Input: part model. Units: mm. Frame: model coordinates. Coordinates: 2 decimals unless noted, no trailing zeros. Write each loop counter-clockwise with the first axis right and the second up, starting at its lowest first coordinate (ties: lowest second). Pieces come first, ordered by that corner, then holes. Notation, with made-up numbers: M 20,66 L 34,66 A21 cw 34,96 Z; hole C 19.5,50 d8. An arc over 180 degrees is marked long. Write each question's results on one line, items separated by ' | '. Start each with the question number.
1. Pull-direction query (Y, two-part tool) for faces 1 (the cylindrical face through (47.53, -9.94, 0.63)), 2 (the cylindrical face through (79.52, -0.45, 0.64)), 3 (the cylindrical face through (79.55, -29.52, 0.64)); classes: +Y half, -Y half, draft (parallel to the pull), parting line (faces both ways), or undercut.
2. Section query D-D, the plane y = -3.75. Output: boundary loops of the cut face in (x, z), and give its area (3 significant figures).
3. Section query C-C, the plane y = -23.5. Output: boundary loops of the cut face in (x, z).
4. First-contact query: pin 1 (1.4 mm diameter, centred on x = 29, y = -26.225, fed in from +Z). Flat tip, straight axial feed; report the tip coordinate or a pass-through.
5. Section query B-B, the plane x = 62. Output: boundary loops of the cut face in (y, z).
6. Section query A-A, the plane x = 31. Output: boundary loops of the cut face in (y, z), and give its area (3 significant figures).
7. Ray query, probe 1 along Y at (x, z) = (73, 0.95); probe 2 along X at (y, z) = (-4.5, 0.25); probe 3 along Y at (x, z) = (40, 0.35). Return the intervals inside material, ascending.
```python
from build123d import *

# Parameters (mm, degrees)
SKETCH1_R           = 1.1303
SKETCH1_R_2         = 1.4732
BOSS_EXTRUDE1_DEPTH = 1.27
FILLET1_R           = 1.5875


with BuildPart() as part:
    # Sketch1 → Boss-Extrude1 (new body)
    with BuildSketch(Plane.XY):
        Polygon((23, 0), (0, 0), (0, -30), (23, -30), (23, -25), (24, -25), (24, -30), (35, -30), (35, -17.3), (45, -17.3), (45, -30), (56, -30), (56, -25), (57, -25), (57, -30), (80, -30), (80, 0), (57, 0), (57, -5), (56, -5), (56, 0), (24, 0), (24, -5), (23, -5), align=None)
        with Locations((7, -26.225)):
            Circle(SKETCH1_R, mode=Mode.SUBTRACT)
        with Locations((18, -26.225)):
            Circle(SKETCH1_R, mode=Mode.SUBTRACT)
        with Locations((29, -26.225)):
            Circle(SKETCH1_R, mode=Mode.SUBTRACT)
        with Locations((51, -26.225)):
            Circle(SKETCH1_R, mode=Mode.SUBTRACT)
        with Locations((62, -26.225)):
            Circle(SKETCH1_R, mode=Mode.SUBTRACT)
        with Locations((73, -26.225)):
            Circle(SKETCH1_R, mode=Mode.SUBTRACT)
        with Locations((7, -11.525)):
            Circle(SKETCH1_R, mode=Mode.SUBTRACT)
        with Locations((18, -11.525)):
            Circle(SKETCH1_R, mode=Mode.SUBTRACT)
        with Locations((31, -10)):
            Circle(SKETCH1_R_2, mode=Mode.SUBTRACT)
        with Locations((40, -11.525)):
            Circle(SKETCH1_R, mode=Mode.SUBTRACT)
        with Locations((49, -10)):
            Circle(SKETCH1_R_2, mode=Mode.SUBTRACT)
        with Locations((62, -11.525)):
            Circle(SKETCH1_R, mode=Mode.SUBTRACT)
        with Locations((73, -11.525)):
            Circle(SKETCH1_R, mode=Mode.SUBTRACT)
    extrude(amount=BOSS_EXTRUDE1_DEPTH)

    # Fillet1
    fillet1_edges = [part.edges().sort_by_distance(p)[0] for p in [
        (0, -30, 0.635),
        (0, 0, 0.635),
        (80, 0, 0.635),
        (80, -30, 0.635),
    ]]
    fillet(fillet1_edges, radius=FILLET1_R)


solid = part.part
```
Answer:
1) face 1: undercut | face 2: +Y half | face 3: -Y half
2) outline: M 0,0 L 23,0 L 23,1.27 L 0,1.27 Z; M 24,0 L 56,0 L 56,1.27 L 24,1.27 Z; M 57,0 L 80,0 L 80,1.27 L 57,1.27 Z | area: 99.1 mm^2
3) outline: M 0,0 L 35,0 L 35,1.27 L 0,1.27 Z; M 45,0 L 80,0 L 80,1.27 L 45,1.27 Z
4) pin 1: through
5) outline: M -30,0 L -27.36,0 L -27.36,1.27 L -30,1.27 Z; M -25.09,0 L -12.66,0 L -12.66,1.27 L -25.09,1.27 Z; M -10.39,0 L 0,0 L 0,1.27 L -10.39,1.27 Z
6) outline: M -30,0 L -11.47,0 L -11.47,1.27 L -30,1.27 Z; M -8.53,0 L 0,0 L 0,1.27 L -8.53,1.27 Z | area: 34.4 mm^2
7) probe 1: -30 to -27.36, -25.09 to -12.66, -10.39 to 0 | probe 2: 0 to 23, 24 to 56, 57 to 80 | probe 3: -17.3 to -12.66, -10.39 to 0
